```python
from build123d import *

# Parameters (mm, degrees)
SKETCH2_W           = 23
SKETCH2_H           = 16
BOSS_EXTRUDE1_DEPTH = 11.5
CUT_EXTRUDE1_DEPTH  = 21.5
CHAMFER1_SIZE       = 0.5
SKETCH4_R           = 1
CUT_EXTRUDE2_DEPTH  = 56


with BuildPart() as part:
    # Sketch1 → Revolve1 (revolve)
    with BuildSketch(Plane.XY, mode=Mode.PRIVATE) as revolve1_sk:
        Polygon((5.807089278, 12.7), (-2.192910722, 12.7), (-2.192910722, 9), (-0.192910722, 9), (-0.192910722, 3), (-2.192910722, 3), (-2.192910722, 0), (1.617747359, 0), (1.617747359, -1.380952381), (-2.192910722, -1.380952381), (-2.192910722, -2.619047619), (1.617747359, -2.619047619), (1.617747359, -4), (-5.342910722, -4), (-5.342910722, -5.238095238), (1.617747359, -5.238095238), (1.617747359, -6.476190476), (-5.342910722, -6.476190476), (-5.342910722, -7.714285714), (1.617747359, -7.714285714), (1.617747359, -8.952380952), (-5.342910722, -8.952380952), (-5.342910722, -10.19047619), (1.617747359, -10.19047619), (1.617747359, -11.428571429), (-5.342910722, -11.428571429), (-5.342910722, -12.666666667), (1.617747359, -12.666666667), (1.617747359, -13.904761905), (-5.342910722, -13.904761905), (-5.342910722, -15.142857143), (1.617747359, -15.142857143), (1.617747359, -16.380952381), (-5.342910722, -16.380952381), (-5.342910722, -17.619047619), (1.617747359, -17.619047619), (1.617747359, -18.857142857), (-5.342910722, -18.857142857), (-5.342910722, -20.095238095), (1.617747359, -20.095238095), (1.617747359, -21.333333333), (-5.342910722, -21.333333333), (-5.342910722, -22.571428571), (1.617747359, -22.571428571), (1.617747359, -23.80952381), (-5.342910722, -23.80952381), (-5.342910722, -25.047619048), (1.617747359, -25.047619048), (1.617747359, -26.285714286), (-5.342910722, -26.285714286), (-5.342910722, -27.523809524), (1.617747359, -27.523809524), (1.617747359, -28.761904762), (-5.342910722, -28.761904762), (-5.342910722, -30), (4.407089278, -30), (4.407089278, -32.1), (5.807089278, -32.1), (5.807089278, -23.767155517), align=None)
    revolve(revolve1_sk.sketch.rotate(Axis((5.807089278, 12.7, 0), (0, -1, 0)), 270), axis=Axis((5.807089278, 12.7, 0), (0, -1, 0)))

    # Sketch2 → Boss-Extrude1 (add)
    with BuildSketch(Plane.XZ.offset(32.1)):
        with Locations((9.307089278, 0)):
            Rectangle(SKETCH2_W, SKETCH2_H)
    extrude(amount=BOSS_EXTRUDE1_DEPTH)

    # Sketch3 → Cut-Extrude1 (cut)
    with BuildSketch(Plane(origin=(0, 0, -8), x_dir=(-1, 0, 0), z_dir=(0, 0, -1))):
        with BuildLine():
            Line((-20.807089278, -38.6), (-20.807089278, -40.6))
            Line((-20.807089278, -40.6), (-15.135516403, -40.6))
            ThreePointArc((-15.135516403, -40.6), (-15.307089278, -39.6), (-15.135516403, -38.6))
            Line((-15.135516403, -38.6), (-20.807089278, -38.6))
        make_face()
        with BuildLine():
            ThreePointArc((-15.135516403, -38.6), (-15.307089278, -39.6), (-15.135516403, -40.6))
            Line((-15.135516403, -40.6), (-12.923340637, -40.6))
            Line((-12.923340637, -40.6), (-12.923340637, -38.6))
            Line((-12.923340637, -38.6), (-15.135516403, -38.6))
        make_face()
        with BuildLine():
            Line((-12.923340637, -40.6), (-15.135516403, -40.6))
            ThreePointArc((-15.135516403, -40.6), (-11.799783342, -42.556795679), (-9.307089278, -39.6))
            ThreePointArc((-9.307089278, -39.6), (-11.799783342, -36.643204321), (-15.135516403, -38.6))
            Line((-15.135516403, -38.6), (-12.923340637, -38.6))
            Line((-12.923340637, -38.6), (-12.923340637, -40.6))
        make_face()
    extrude(amount=-CUT_EXTRUDE1_DEPTH, mode=Mode.SUBTRACT)

    # Chamfer1
    chamfer1_edges = [part.edges().sort_by_distance(p)[0] for p in [
        (5.807089278, -32.1, -1.4),
        (-2.192910722, -32.1, 0),
        (-2.192910722, -37.85, 8),
        (9.307089278, -32.1, -8),
        (-2.192910722, -37.85, -8),
        (20.807089278, -32.1, 0),
        (20.807089278, -42.1, -8),
        (9.307089278, -32.1, 8),
        (20.807089278, -42.1, 8),
        (-2.192910722, -43.6, 0),
        (9.307089278, -43.6, -8),
        (20.807089278, -43.6, 0),
        (9.307089278, -43.6, 8),
        (20.807089278, -35.35, 8),
        (20.807089278, -35.35, -8),
    ]]
    chamfer(chamfer1_edges, length=CHAMFER1_SIZE)

    # Sketch4 → Cut-Extrude2 (cut)
    with BuildSketch(Plane(origin=(0, 12.7, 0), x_dir=(1, 0, 0), z_dir=(0, 1, 0))):
        with Locations(Location((5.807089278, 0, 0), (0, 0, 180))):
            Circle(SKETCH4_R)
    extrude(amount=-CUT_EXTRUDE2_DEPTH, mode=Mode.SUBTRACT)


solid = part.part
```
Geometry: final body of the model. Coordinates: model frame, mm. A direction names the side the tool comes from. Give positions to 0.01 mm unless a question says otherwise; leave off trailing zeros. Loops run counter-clockwise (first coordinate to the right, second up) from the corner with the lowest first, then second, coordinate; pieces in that order, holes last. Notation, with made-up numbers: (-14.75, -20) -> (2.25, -20) arc R23 ccw to (2.25, 13) -> close; hole circle Ø11 at (57, 54). An arc over 180 degrees is marked (long way). Use one line per item in the form item = value.
Item 1: Pin query (flat end, axial travel): P1, Ø8, axis at x = 12, y = -31, coming from the -Z side; P2, Ø8, axis at y = -5, z = -4.5, coming from the +X side; P3, Ø1, axis at x = -2.5, z = -4.5, coming from the -Y side; P4, Ø5, axis at y = -32.5, z = -3, coming from the +X side. Return the tip coordinate at first contact, or that it passes through.
A:
P1 = -10.91
P2 = 16.95
P3 = -43.29
P4 = 20.81
Item 2: Line query: probe 1 along Y at (x, z) = (4.75, -2.75); probe 2 along Y at (x, z) = (19.75, 2.5); probe 3 along X at (y, z) = (9.5, -0.5). Output: solid intervals per line, ascending.
A:
probe_1 = -43.6 to -32.1, -30 to 12.7
probe_2 = -43.6 to -40.6, -38.6 to -32.1
probe_3 = -2.18 to 4.94, 6.67 to 13.79
Item 3: Section query B-B on y = 6. Output: boundary loops of the cut face in (x, z), and give its area (3 significant figures).
A:
outline = circle Ø12 at (5.81, 0); hole circle Ø2 at (5.81, 0)
area = 110 mm^2
Item 4: Section query A-A on x = 17.75. Output: boundary loops of the cut face in (y, z), and give its area (4 significant figures).
A:
outline = (-43.6, -7.5) -> (-43.1, -8) -> (-40.6, -8) -> (-40.6, 8) -> (-43.1, 8) -> (-43.6, 7.5) -> close; (-38.6, -8) -> (-32.6, -8) -> (-32.1, -7.5) -> (-32.1, 7.5) -> (-32.6, 8) -> (-38.6, 8) -> close
area = 151.5 mm^2
Item 5: Access query for faces 1 (the face through (11, -16.381, 0)), 2 (the face through (9, -38, 8)), 3 (the face through (-3.595, -7.104, 5.994)). Directions: +Z, -Z, +X, -X, +Y, -Y. A direction counts if a zero-diameter tool reaches every point of the face in a straight line with its end or side. Return the directions, or none.
A:
face_1 = none
face_2 = +Z, +X, -X, -Y
face_3 = +Y
